Input: part model. Units: mm. Frame: model coordinates. Face numbers are marked on the shaded views. Round coordinates to 2 decimals unless told otherwise and drop trailing zeros. Order: outer loops, then holes, each group sorted by start corner. A loop starts at its lowest first (then second) coordinate and runs counter-clockwise, first axis right, second up. Notation, with made-up numbers: (37, 31.5) -> (96, 31.5) arc R28 cw to (96, 51.5) -> close; hole circle Ø6 at (-14.75, 58). An arc over 180 degrees is marked (long way). Answer as CSV lines item,"result". Start each with the question number.
1) Section query B-B, the plane z = 387. Output: boundary loops of the cut face in (x, y).
2) Mould query, pull axis Z, two halves, no side actions, for the marked faces 1 and 2. Classes: +Z half, -Z half, draft (parallel to the pull), parting line (faces both ways), or undercut.
3) Section query C-C, the plane x = -37. Output: boundary loops of the cut face in (y, z).
4) Section query A-A, the plane y = -1. Output: boundary loops of the cut face in (x, z) (3 decimals).
5) Line query: L1, parallel to Z at x = 17.5, y = -1.5 (3 decimals); L2, parallel to Y at x = 0, z = 643; L3, parallel to X at y = 0, z = 414. Output: solid intervals per line, ascending.
6) First-contact query: P1, Ø11.5, axis at x = 33, y = 2, coming from the -Z side; P2, Ø19, axis at x = 26.5, y = -9, coming from the +Z side; P3, Ø11.5, axis at y = 4, z = 47, coming from the +X side. Flat tips, straight axial feed; report the tip coordinate or a pass-through.
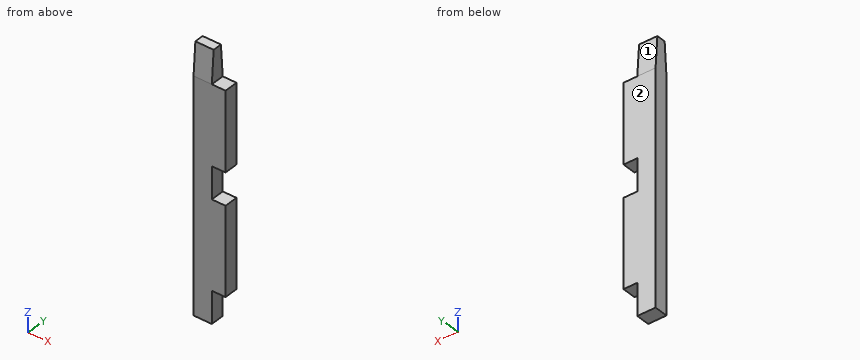
```python
from build123d import *

# Parameters (mm, degrees)
F0_W     = 88.9
F0_H     = 38.1
F1_DEPTH = 730.25
F2_W     = 38.1
F2_H     = 88.9
F3_DEPTH = 38.101
F5_DEPTH = 50.801


with BuildPart() as f1:
    # F0 (on Top) → F1 (new body)
    with BuildSketch(Plane.XY):
        Rectangle(F0_W, F0_H)
    extrude(amount=F1_DEPTH)

    # F2 (on face) → F3 (cut, through all)
    with BuildSketch(Plane.XZ.offset(19.05)):
        with Locations((25.4, 44.45)):
            Rectangle(F2_W, F2_H)
        with Locations((25.4, 377.825)):
            Rectangle(F2_W, F2_H)
        with Locations((25.4, 685.8)):
            Rectangle(F2_W, F2_H)
    extrude(amount=-F3_DEPTH, mode=Mode.SUBTRACT)

    # F4 (on face) → F5 (cut, through all)
    with BuildSketch(Plane.YZ.offset(6.35)):
        Polygon((-12.7, 730.25), (-19.05, 730.25), (-19.05, 641.35), align=None)
        Polygon((19.05, 641.35), (19.05, 730.25), (12.7, 730.25), align=None)
    extrude(amount=-F5_DEPTH, mode=Mode.SUBTRACT)


solid = f1.part
```
Findings:
1,outline,"(-44.45, -19.05) -> (6.35, -19.05) -> (6.35, 19.05) -> (-44.45, 19.05) -> close"
2,face 1,"+Z half"
2,face 2,"draft"
3,outline,"(-19.05, 0) -> (19.05, 0) -> (19.05, 641.35) -> (12.7, 730.25) -> (-12.7, 730.25) -> (-19.05, 641.35) -> close"
4,outline,"(-44.45, 0) -> (6.35, 0) -> (6.35, 88.9) -> (44.45, 88.9) -> (44.45, 333.375) -> (6.35, 333.375) -> (6.35, 422.275) -> (44.45, 422.275) -> (44.45, 641.35) -> (6.35, 641.35) -> (6.35, 730.25) -> (-44.45, 730.25) -> close"
5,L1,"z = 88.9 to 333.375, 422.275 to 641.35"
5,L2,"y = -18.93 to 18.93"
5,L3,"x = -44.45 to 6.35"
6,P1,"stops at z = 88.9"
6,P2,"stops at z = 641.35"
6,P3,"stops at x = 6.35"
